Verification items for the finished model (mm, model axes). Give positions to 0.01 mm unless a question says otherwise; leave off trailing zeros. Loops run counter-clockwise (first coordinate to the right, second up) from the corner with the lowest first, then second, coordinate; pieces in that order, holes last. Notation, with made-up numbers: M 77,-4.75 L 85,-4.75 A10 cw 85,0.25 Z; hole C 74,31.5 d9. An arc over 180 degrees is marked long. Answer in a Markdown table with one row per item.
```python
from build123d import *

# Parameters (mm, degrees)
BOSS_EXTRUDE1_DEPTH              = 6
F_10_0MM_DOWEL_HOLE2_D           = 10
F_10_0MM_DOWEL_HOLE2_DEPTH       = 50
F_10_0MM_DOWEL_HOLE2_CSINK_D     = 10.05
F_10_0MM_DOWEL_HOLE2_CSINK_ANGLE = 90
F_10_0MM_DOWEL_HOLE2_TIP         = 3.004303095


with BuildPart() as part:
    # Sketch1 → Boss-Extrude1 (new body)
    with BuildSketch(Plane.XY):
        Polygon((-47.927135712, -8.080790765), (13.552864288, -8.080790765), (61.932230114, 57.778577521), (40.312864288, 110.519482152), (-74.687135712, 110.519482152), (-94.182283881, 56.957002767), align=None)
    extrude(amount=BOSS_EXTRUDE1_DEPTH)

    # Ø10.0mm Dowel Hole2
    with Locations(Plane.XY.offset(6)):
        with Locations((-16.890604688, 62.873141165)):
            CounterSinkHole(F_10_0MM_DOWEL_HOLE2_D / 2, F_10_0MM_DOWEL_HOLE2_CSINK_D / 2, depth=F_10_0MM_DOWEL_HOLE2_DEPTH, counter_sink_angle=F_10_0MM_DOWEL_HOLE2_CSINK_ANGLE)
            with Locations((0, 0, -(F_10_0MM_DOWEL_HOLE2_DEPTH + F_10_0MM_DOWEL_HOLE2_TIP / 2))):  # 118° drill point
                Cone(0, F_10_0MM_DOWEL_HOLE2_D / 2, F_10_0MM_DOWEL_HOLE2_TIP, mode=Mode.SUBTRACT)


solid = part.part
```
Item 1: Sectioned sample at B-B (x = 17.5). Record the cut outline in (y, z).
Reported:
| item | result |
|---|---|
| outline | M -2.71,0 L 110.52,0 L 110.52,6 L -2.71,6 Z |
Item 2: Go/stop test with flat-tipped pins: pin 1 (1.5 mm diameter, centred on x = -52.5, z = 4.5, fed in from -Y); pin 2 (6 mm diameter, centred on x = -16.89, y = 62.87, fed in from +Z). Record where each tip stops, or that it passes through.
Reported:
| item | result |
|---|---|
| pin 1 | stops at y = -2.71 |
| pin 2 | passes through |
Item 3: Release check for a two-part mould opening along X. For faces 1 (the flat face through (-18, -8.081, 3)), 2 (the flat face through (-84.3, 84.11, 2.96)), 3 (the flat face through (37.404, 24.388, 2.958)), 4 (the cylindrical face through (-13.205, 66.252, 2.946)) record: released by +X, released by -X, zero draft, split by the parting line, or undercut.
Reported:
| item | result |
|---|---|
| face 1 | zero draft |
| face 2 | released by -X |
| face 3 | released by +X |
| face 4 | undercut |
Item 4: Sectioned sample at C-C (y = 34.5). Record the cut outline in (x, z).
Reported:
| item | result |
|---|---|
| outline | M -78.21,0 L 44.83,0 L 44.83,6 L -78.21,6 Z |
Item 5: Scan lines: L1, parallel to Y at x = -13, z = 0.95; L2, parallel to X at y = 105, z = 2; L3, parallel to X at y = 101, z = 2.4. Record each from-to range of solid material in increasing order. Write a range as [from, to].
Reported:
| item | result |
|---|---|
| L1 | y = [-8.08, 59.73], [66.01, 110.52] |
| L2 | x = [-76.7, 42.58] |
| L3 | x = [-78.15, 44.22] |
Item 6: Sectioned sample at A-A (z = 1.6). Record the cut outline in (x, y), and give its area (3 significant figures).
Reported:
| item | result |
|---|---|
| outline | M -94.18,56.96 L -47.93,-8.08 L 13.55,-8.08 L 61.93,57.78 L 40.31,110.52 L -74.69,110.52 Z; hole C -16.89,62.87 d10 |
| area | 14,200 mm^2 |
